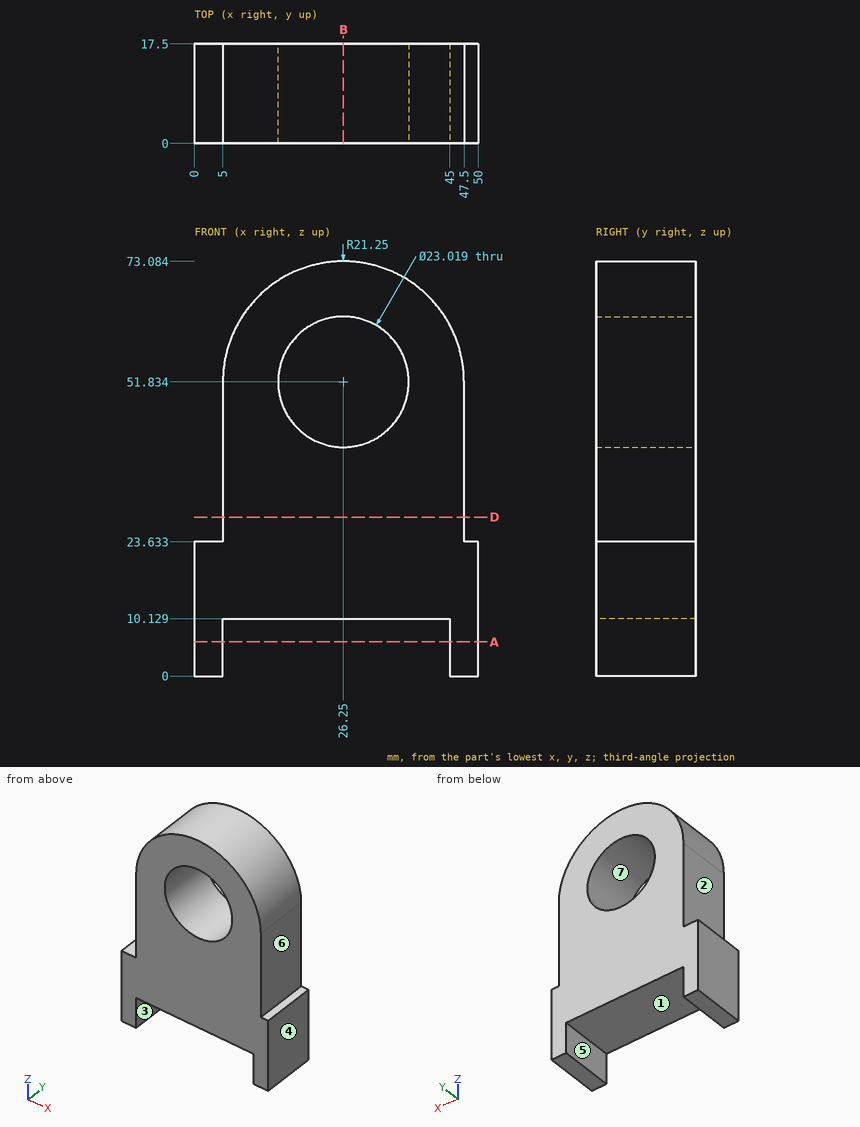
Design review of the part shown in the three views and the two pictorial views. Dimensions are in mm from the part's minimum x, y and z. A direction names the side the tool comes from. Coordinates: 2 decimals unless noted, no trailing zeros. Loops run counter-clockwise (first coordinate to the right, second up) from the corner with the lowest first, then second, coordinate; pieces in that order, holes last. Notation, with made-up numbers: (8, -12) -> (36, -12) arc R25 cw to (36, 7) -> close; hole circle Ø9 at (-34, 70.25). An arc over 180 degrees is marked (long way). Answer as CSV lines item,"result".
Item 1: Draft analysis for pull direction X (two halves, no side actions). For the marked faces 1, 2, 3 and 4, state which applies: +X half, -X half, draft (parallel to the pull), parting line (faces both ways), or undercut.
Results below:
face 1,"undercut"
face 2,"-X half"
face 3,"undercut"
face 4,"+X half"
Item 2: Take a section at D-D, the plane z = 28. State the section outline as (x, y) points, and give its area (3 significant figures).
Results below:
outline,"(5, 0) -> (47.5, 0) -> (47.5, 17.5) -> (5, 17.5) -> close"
area,"744 mm2"
Item 3: For L1, parallel to Z at x = 26.25, y = 7.75 (1 decimal); L2, parallel to X at y = 2.25, z = 8.5; L3, parallel to X at y = 12.75, z = 55 (1 decimal), list the stretches that pass through material, from the lowest coordinate up.
Results below:
L1,"z = 10.1 to 40.3, 63.3 to 73.1"
L2,"x = 0 to 5, 45 to 50"
L3,"x = 5.2 to 15.2, 37.3 to 47.3"
Item 4: Take a section at A-A, the plane z = 6. State the section outline as (x, y) points.
Results below:
outline,"(0, 0) -> (5, 0) -> (5, 17.5) -> (0, 17.5) -> close; (45, 0) -> (50, 0) -> (50, 17.5) -> (45, 17.5) -> close"
Item 5: Machinability: for the marked faces 5, 6 and 7, which of the approach directions +Z, -Z, +X, -X, +Y, -Y give a long, thin tool a straight path to every point of the face, cutting with its end or side? Answer none if there is none.
Results below:
face 5,"-Z, +Y, -Y"
face 6,"+Z, +X, +Y, -Y"
face 7,"+Y, -Y"
Item 6: Insertion check: pin 1 (3 mm diameter, centred on y = 7, z = 4, fed in from -X); pin 2 (4 mm diameter, centred on y = 7, z = 56.5, fed in from +X); pin 3 (1.5 mm diameter, centred on x = 2.5, y = 12.5, fed in from +Z); pin 4 (1 mm diameter, centred on y = 10, z = 44.5, fed in from -X). Each pin has a flat end and moves straight along its axis. Give the tip position at first contact, or say it passes through.
Results below:
pin 1,"stops at x = 0"
pin 2,"stops at x = 47.33"
pin 3,"stops at z = 23.63"
pin 4,"stops at x = 5"
Item 7: Take a section at B-B, the plane x = 26.25. State the section outline as (y, z) points (1 decimal), and give its area (3 significant figures).
Results below:
outline,"(0, 10.1) -> (17.5, 10.1) -> (17.5, 40.3) -> (0, 40.3) -> close; (0, 63.3) -> (17.5, 63.3) -> (17.5, 73.1) -> (0, 73.1) -> close"
area,"699 mm2"
